from build123d import *

# Parameters (mm, degrees)
SKETCH2_W                     = 12.7
SKETCH2_H                     = 109
BOSS_EXTRUDE1_DEPTH           = 12.7
SKETCH5_W                     = 12.7
SKETCH5_H                     = 29
BOSS_EXTRUDE2_DEPTH           = 5
CBORE_FOR_M5_SHCS1_AT_2_COUNT = 2
CBORE_FOR_M5_SHCS1_AT_2_PITCH = 15
CHAMFER1_SIZE                 = 5
SKETCH7_W                     = 12.7
SKETCH7_H                     = 12.7
BOSS_EXTRUDE4_DEPTH           = 34.05
SKETCH9_W                     = 12.7
SKETCH9_H                     = 12.7
CUT_EXTRUDE2_DEPTH            = 6.35
SKETCH6_R                     = 2.5
BOSS_EXTRUDE7_DEPTH           = 10
CHAMFER3_SIZE                 = 6.35


with BuildPart() as part:
    # Sketch2 → Boss-Extrude1 (new body)
    with BuildSketch(Plane(origin=(0, 0, 0), x_dir=(1, 0, 0), z_dir=(0, 1, 0))):
        Rectangle(SKETCH2_W, SKETCH2_H)
    extrude(amount=BOSS_EXTRUDE1_DEPTH)

    # Sketch5 → Boss-Extrude2 (add)
    with BuildSketch(Plane(origin=(0, 12.7, 0), x_dir=(1, 0, 0), z_dir=(0, 1, 0))):
        with Locations((0, 40)):
            Rectangle(SKETCH5_W, SKETCH5_H)
    extrude(amount=BOSS_EXTRUDE2_DEPTH)

    # Sketch4 → CBORE for M5 SHCS1 (revolve, cut)
    with BuildSketch(Plane(origin=(0, 0, -47.5), x_dir=(0, 0, -1), z_dir=(1, 0, 0))):
        Polygon((0, 0), (0, 17.7), (2.9, 17.7), (2.9, 5), (5, 5), (5, 0.020977491), (5.025, 0), align=None)
    cbore_for_m5_shcs1 = revolve(axis=Axis((0, -6.35, -47.5), (0, 1, 0)), mode=Mode.SUBTRACT)

    # CBORE for M5 SHCS1 at 2: CBORE for M5 SHCS1 ×2
    with Locations(*[(0, 0, i * CBORE_FOR_M5_SHCS1_AT_2_PITCH) for i in range(1, CBORE_FOR_M5_SHCS1_AT_2_COUNT)]):
        add(cbore_for_m5_shcs1, mode=Mode.SUBTRACT)

    # Chamfer1
    chamfer1_edges = [part.edges().sort_by_distance(p)[0] for p in [
        (0, 12.7, -25.5),
    ]]
    chamfer(chamfer1_edges, length=CHAMFER1_SIZE - 0.0001)  # a hair under: the kernel refuses the full size

    # Sketch7 → Boss-Extrude4 (add)
    with BuildSketch(Plane(origin=(0, 12.7, 0), x_dir=(1, 0, 0), z_dir=(0, 1, 0))):
        with Locations((0, -48.15)):
            Rectangle(SKETCH7_W, SKETCH7_H)
    extrude(amount=BOSS_EXTRUDE4_DEPTH)

    # Sketch9 → Cut-Extrude2 (cut)
    with BuildSketch(Plane.XY.offset(54.5)):
        with Locations((0, 40.4)):
            Rectangle(SKETCH9_W, SKETCH9_H)
    extrude(amount=-CUT_EXTRUDE2_DEPTH, mode=Mode.SUBTRACT)

    # Sketch6 → Boss-Extrude7 (add)
    with BuildSketch(Plane.XY.offset(48.15)):
        with Locations((0, 40.4)):
            Circle(SKETCH6_R)
    extrude(amount=BOSS_EXTRUDE7_DEPTH)

    # Chamfer3
    chamfer3_edges = [part.edges().sort_by_distance(p)[0] for p in [
        (0, 34.05, 54.5),
    ]]
    chamfer(chamfer3_edges, length=CHAMFER3_SIZE - 0.0001)  # a hair under: the kernel refuses the full size


solid = part.part
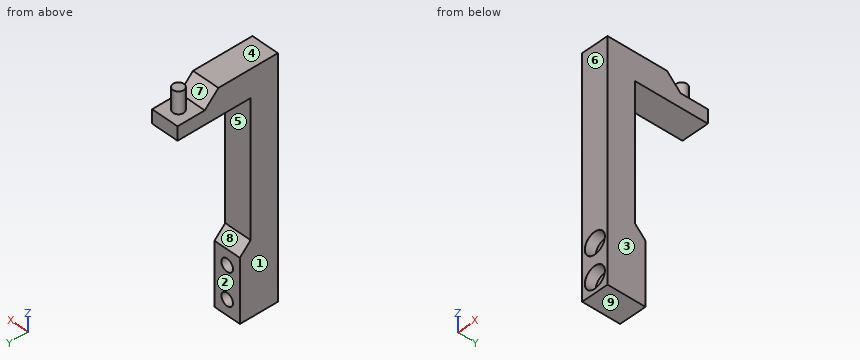
Verification items for the finished model (mm, model axes). Face numbers are marked on the shaded views. A direction names the side the tool comes from. Give positions to 0.01 mm unless a question says otherwise; leave off trailing zeros. Write each loop counter-clockwise with the first axis right and the second up, starting at its lowest first coordinate (ties: lowest second). Pieces come first, ordered by that corner, then holes.
(1) Gauge pin test, flat ends, axial feed: pin 1 (3 mm diameter, centred on x = -2, y = 22.5, fed in from -Z); pin 2 (6.5 mm diameter, centred on x = -0.5, z = -40.5, fed in from +Y); pin 3 (1 mm diameter, centred on x = 2.5, z = 10.5, fed in from +Y). Record the tip position at first contact, or that the pin passes through.
(2) Mould release check, pull along Y, two halves, no side actions. Record for the marked faces 6, 7, 8 and 9: +Y half, -Y half, draft (parallel to the pull), parting line (faces both ways), or undercut.
(3) Access from +Z, -Z, +X, -X, +Y, -Y to the whole of each face (thin tool, end or side, straight path). Record for the marked faces 1, 2, 3, 4 and 5.
(4) Cross-section at B-B (y = 40.4). Enter the section's corners in (x, z).
(5) Material ranges on line 1 (Z direction, x = 0, y = 3.25); line 2 (Z direction, x = 0, y = 9.5); line 3 (X direction, y = 2.85, z = -32.5), recorded low to high.
(6) Cross-section at D-D (z = -22). Enter the section's corners in (x, y), plus the area to 3 significant figures.
(7) Cross-section at A-A (z = -47.5). Enter the section's corners in (x, y) (3 decimals).
(8) Cross-section at C-C (x = 0). State how many separate pieces and enclosed holes the cut face has, plus the area to 3 significant figures.
Worked out:
1. pin 1: stops at z = 41.8
1. pin 2: stops at y = 17.7
1. pin 3: stops at y = 12.7
2. face 6: -Y half
2. face 7: undercut
2. face 8: +Y half
2. face 9: draft
3. face 1: +Z, -Z, -X, +Y, -Y
3. face 2: -Z, +X, -X, +Y
3. face 3: +Z, -Z, +X, +Y, -Y
3. face 4: +Z, +X, -X, -Y
3. face 5: +X, -X, +Y
4. outline: (-6.35, 41.8) - (6.35, 41.8) - (6.35, 48.15) - (2.5, 48.15) - (2.5, 58.15) - (-2.5, 58.15) - (-2.5, 48.15) - (-6.35, 48.15) - close
5. line 1: z = -54.5 to -52.5, -42.5 to -37.5, -27.5 to 54.5
5. line 2: z = -54.5 to -50.4, -44.6 to -35.4, -29.6 to 54.5
5. line 3: x = -6.35 to -5, 5 to 6.35
6. outline: (-6.35, 0) - (6.35, 0) - (6.35, 14.2) - (-6.35, 14.2) - close
6. area: 180 mm2
7. outline: (-6.35, 0) - (-5.025, 0) - (-5, 0.021) - (-5, 5) - (-2.9, 5) - (-2.9, 17.7) - (-6.35, 17.7) - close; (2.9, 5) - (5, 5) - (5, 0.021) - (5.025, 0) - (6.35, 0) - (6.35, 17.7) - (2.9, 17.7) - close
8. separate pieces: 3
8. enclosed holes: 0
8. area: 1,680 mm2
